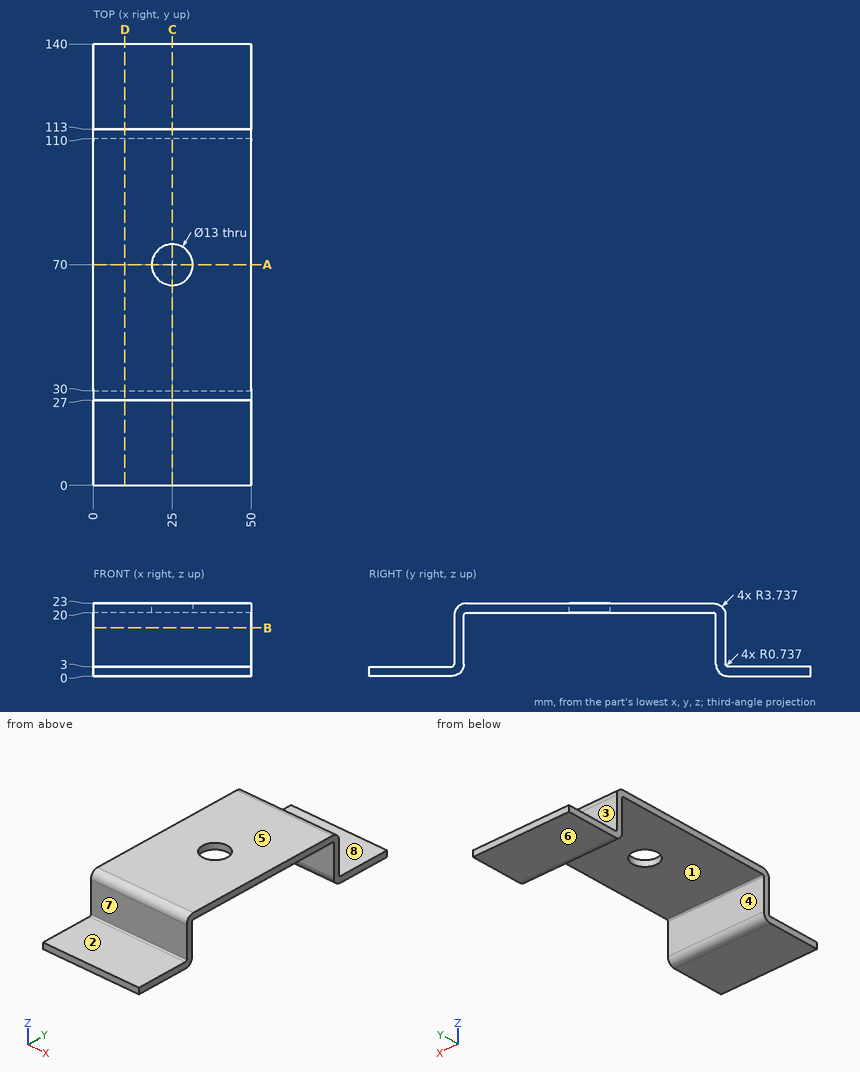
Could you check a few things on this drawing? It's one solid part, dimensions in mm from its lowest x, y, z. A direction names the side the tool comes from. Give positions to 0.01 mm unless a question says otherwise; leave off trailing zeros. Loops run counter-clockwise (first coordinate to the right, second up) from the corner with the lowest first, then second, coordinate; pieces in that order, holes last. Notation, with made-up numbers: (-10.5, -37.5) -> (35.5, -37.5) arc R27 cw to (35.5, 1.5) -> close; hole circle Ø7 at (32.5, 8.25). An arc over 180 degrees is marked (long way). Use one line per item in the form item = value. Start each with the question number.
1) Please list where these lines run through material, in increasing order: line 1 along Y through (x, z) = (10, 16); line 2 along Z through (x, y) = (17, 54); line 3 along Y through (x, z) = (25, 22.05) (1 decimal).
2) Imagine slicing it at A-A (y = 70). Please give me the cut outline in (x, z), then the cut area to 3 significant figures.
3) For P1, Ø8, axis at x = 23, z = 10.5, coming from the +Y side; P2, Ø25, axis at x = 34.5, y = 81, coming from the -Z side; P3, Ø12.5, axis at x = 30.5, z = 13.5, coming from the -Y side; P4, Ø6, axis at y = 90, z = 19.5, coming from the +X side, each with a flat end and sliding along its axis, tell me the tip position at first contact or that it passes through.
4) Thinking about a two-plate mould opening in Y: for the marked faces 1, 2 and 3, which applies, +Y half, -Y half, draft (parallel to the pull), parting line (faces both ways), or undercut?
5) Imagine slicing it at C-C (x = 25). Please give me the cut outline in (y, z).
6) Which directions (+Z, -Z, +X, -X, +Y, -Y) give clear straight access to the entire face, cutting with the end or side of a thin tool? Please do the marked faces 4, 5, 6, 7 and 8.
7) Imagine slicing it at B-B (z = 15.25). Please give me the cut outline in (x, y).
8) Imagine slicing it at D-D (x = 10). Please give me the cut outline in (y, z).
Check values:
q1.line_1 = 27 to 30, 110 to 113
q1.line_2 = 20 to 23
q1.line_3 = 28.2 to 63.5, 76.5 to 111.8
q2.outline = (0, 20) -> (18.5, 20) -> (18.5, 23) -> (0, 23) -> close; (31.5, 20) -> (50, 20) -> (50, 23) -> (31.5, 23) -> close
q2.area = 111 mm^2
q3.P1 = 113
q3.P2 = 20
q3.P3 = 27
q3.P4 = 50
q4.face_1 = undercut
q4.face_2 = draft
q4.face_3 = +Y half
q5.outline = (0, 0) -> (26.26, 0) arc R3.74 ccw to (30, 3.74) -> (30, 19.26) arc R0.74 cw to (30.74, 20) -> (63.5, 20) -> (63.5, 23) -> (30.74, 23) arc R3.74 ccw to (27, 19.26) -> (27, 3.74) arc R0.74 cw to (26.26, 3) -> (0, 3) -> close; (76.5, 20) -> (109.26, 20) arc R0.74 cw to (110, 19.26) -> (110, 3.74) arc R3.74 ccw to (113.74, 0) -> (140, 0) -> (140, 3) -> (113.74, 3) arc R0.74 cw to (113, 3.74) -> (113, 19.26) arc R3.74 ccw to (109.26, 23) -> (76.5, 23) -> close
q6.face_4 = -Z, +X, -X
q6.face_5 = +Z, +X, -X, +Y, -Y
q6.face_6 = -Z, +X, -X, +Y, -Y
q6.face_7 = +Z, +X, -X, -Y
q6.face_8 = +Z, +X, -X, +Y
q7.outline = (0, 27) -> (50, 27) -> (50, 30) -> (0, 30) -> close; (0, 110) -> (50, 110) -> (50, 113) -> (0, 113) -> close
q8.outline = (0, 0) -> (26.26, 0) arc R3.74 ccw to (30, 3.74) -> (30, 19.26) arc R0.74 cw to (30.74, 20) -> (109.26, 20) arc R0.74 cw to (110, 19.26) -> (110, 3.74) arc R3.74 ccw to (113.74, 0) -> (140, 0) -> (140, 3) -> (113.74, 3) arc R0.74 cw to (113, 3.74) -> (113, 19.26) arc R3.74 ccw to (109.26, 23) -> (30.74, 23) arc R3.74 ccw to (27, 19.26) -> (27, 3.74) arc R0.74 cw to (26.26, 3) -> (0, 3) -> close
